Can you work these out from the model? Positions are in its coordinate system, mm. Round coordinates to 2 decimals unless told otherwise and drop trailing zeros. Write each loop counter-clockwise with the first axis right and the second up, starting at its lowest first coordinate (ties: lowest second). Pieces come first, ordered by that corner, then holes. Notation, with made-up numbers: M 54.5,84 L 95.5,84 A25 ccw 95.5,96 Z; hole C 44.25,15.5 d4. An arc over 180 degrees is marked long. Answer as a JSON object with one key per item and string values. Group by question number.
1) Please list where these lines run through material, in increasing order: L1, parallel to X at y = 24, z = 6; L2, parallel to X at y = 7, z = 9.5; L3, parallel to Z at x = -33, y = 29. Write a range as [from, to].
2) Suppose I cut it at B-B, the plane y = -11. Write out the boundary of the cut face in (x, z), and give its area (3 significant figures).
3) If we mould it in two halves opening along X, with no side actions, what happens to faces 1 (the cylindrical face through (-22.267, 13.588, 9.053)), 2 (the cylindrical face through (-19, -15, 9))? For each: +X half, -X half, draft (parallel to the pull), parting line (faces both ways), or undercut.
4) I'm going to push a flat-ended pin straight in: pin 1 Ø6 at (x, z) = (-3.5, 7) entering from +Y. Where does the tip first touch, or does it pass through?
5) Suppose I cut it at C-C, the plane z = 6.35. State how many separate pieces and enclosed holes the cut face has, and give its area (3 significant figures).
from build123d import *

# Parameters (mm, degrees)
F0_W     = 38.1
F0_H     = 76.2
F1_DEPTH = 12.7
F2_R     = 4
F3_DEPTH = 38.101
F4_R     = 4
F5_DEPTH = 76.201


with BuildPart() as f1:
    # F0 (on Top) → F1 (new body)
    with BuildSketch(Plane.XY):
        with Locations((-16.005945, -2.513404)):
            Rectangle(F0_W, F0_H)
    extrude(amount=F1_DEPTH)

    # F2 (on face) → F3 (cut, through all)
    with BuildSketch(Plane.YZ.offset(3.044055)):
        with Locations((-34.263404, 6.35)):
            Circle(F2_R)
        with Locations((-21.563404, 6.35)):
            Circle(F2_R)
        with Locations((-8.863404, 6.35)):
            Circle(F2_R)
        with Locations((3.836596, 6.35)):
            Circle(F2_R)
        with Locations((16.536596, 6.35)):
            Circle(F2_R)
        with Locations((29.236596, 6.35)):
            Circle(F2_R)
    extrude(amount=-F3_DEPTH, mode=Mode.SUBTRACT)

    # F4 (on face) → F5 (cut, through all)
    with BuildSketch(Plane.XZ.offset(40.613404)):
        with Locations((-28.705945, 6.35)):
            Circle(F4_R)
        with Locations((-16.005945, 6.35)):
            Circle(F4_R)
        with Locations((-3.305945, 6.35)):
            Circle(F4_R)
    extrude(amount=-F5_DEPTH, mode=Mode.SUBTRACT)


solid = f1.part
Results:
{
 "1": {"L1": "[-35.06, -32.69], [-24.72, -19.99], [-12.02, -7.29], [0.68, 3.04]", "L2": "[-35.06, -31.17], [-26.24, -18.47], [-13.54, -5.77], [-0.84, 3.04]", "L3": "[0, 2.36], [10.34, 12.7]"},
 "2": {"outline": "M -35.06,0 L 3.04,0 L 3.04,2.97 L -1.17,2.97 A4 cw -5.44,2.97 L -13.87,2.97 A4 cw -18.14,2.97 L -26.57,2.97 A4 cw -30.84,2.97 L -35.06,2.97 Z; M -35.06,9.73 L -30.84,9.73 A4 cw -26.57,9.73 L -18.14,9.73 A4 cw -13.87,9.73 L -5.44,9.73 A4 cw -1.17,9.73 L 3.04,9.73 L 3.04,12.7 L -35.06,12.7 Z", "area": "215 mm^2"},
 "3": {"face 1": "draft", "face 2": "undercut"},
 "4": {"pin 1": "through"},
 "5": {"separate pieces": "28", "enclosed holes": "0", "area": "398 mm^2"}
}
